The model under review builds one solid part; all positions refer to its coordinate system, in mm. Give positions to 0.01 mm unless a question says otherwise; leave off trailing zeros. Order: outer loops, then holes, each group sorted by start corner. A loop starts at its lowest first (then second) coordinate and runs counter-clockwise, first axis right, second up. Notation, with made-up numbers: (49.5, 56.5) - (65.5, 56.5) arc R25 cw to (65.5, 85.5) - close; hole circle Ø7 at (49, 64). An arc over 180 degrees is marked (long way). Use CSV: the item, a comma, the result in double quotes.
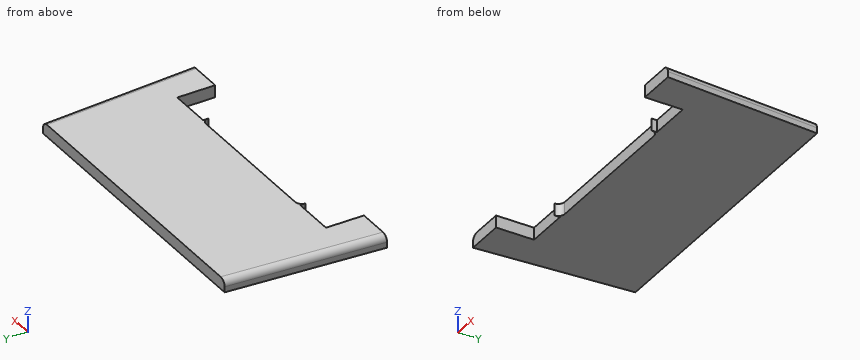
```python
from build123d import *

# Parameters (mm, degrees)
BOSS_EXTRUDE1_DEPTH = 25
FILLET1_R           = 13.5


with BuildPart() as part:
    # Sketch1 → Boss-Extrude1 (new body)
    with BuildSketch(Plane.XY):
        with BuildLine():
            Line((-251.2, -2), (-251.2, -80))
            Line((-251.2, -80), (-329.1, -80))
            Line((-329.1, -80), (-306.723420178, 240))
            Line((-306.723420178, 240), (306.723420178, 240))
            Line((306.723420178, 240), (329.1, -80))
            Line((329.1, -80), (251.2, -80))
            Line((251.2, -80), (251.2, -2))
            Line((251.2, -2), (163.8, -2))
            Line((163.8, -2), (163.8, -13))
            ThreePointArc((163.8, -13), (159.992388155, -3.807611845), (150.8, 0))
            Line((150.8, 0), (-150.8, 0))
            ThreePointArc((-150.8, 0), (-159.992388155, -3.807611845), (-163.8, -13))
            Line((-163.8, -13), (-163.8, -2))
            Line((-163.8, -2), (-251.2, -2))
        make_face()
    extrude(amount=BOSS_EXTRUDE1_DEPTH)

    # Fillet1
    fillet1_edges = [part.edges().sort_by_distance(p)[0] for p in [
        (317.911710089, 80, 25),
        (-317.911710089, 80, 25),
    ]]
    fillet(fillet1_edges, radius=FILLET1_R)


solid = part.part
```
Item 1: Take a section at C-C, the plane x = -210.5. Give the boundary of the cut face in (y, z).
Results list:
outline,"(-2, 0) - (240, 0) - (240, 25) - (-2, 25) - close"
Item 2: Clearance check with flat-ended pins moving along their axes: pin 1 (5 mm diameter, centred on y = 111, z = 15, fed in from -X); pin 2 (3.5 mm diameter, centred on y = -9.5, z = 10.5, fed in from -X); pin 3 (7.5 mm diameter, centred on x = 201.5, z = 16, fed in from -Y). State where each tip first meets the part, or that it passes through.
Results list:
pin 1,"stops at x = -315.77"
pin 2,"stops at x = -324.29"
pin 3,"stops at y = -2"
Item 3: Take a section at A-A, the plane z = 5.75. Give the boundary of the cut face in (x, y).
Results list:
outline,"(-329.1, -80) - (-251.2, -80) - (-251.2, -2) - (-163.8, -2) - (-163.8, -13) arc R13 cw to (-150.8, 0) - (150.8, 0) arc R13 cw to (163.8, -13) - (163.8, -2) - (251.2, -2) - (251.2, -80) - (329.1, -80) - (306.72, 240) - (-306.72, 240) - close"
Item 4: Take a section at B-B, the plane x = 55. Give the boundary of the cut face in (y, z).
Results list:
outline,"(0, 0) - (240, 0) - (240, 25) - (0, 25) - close"
Item 5: Wall thickness on L1, parallel to X at y = -34.5, z = 6.5; L2, parallel to Y at x = -146.5, z = 4.5; L3, parallel to Y at x = -191, z = 9.75: over which ranges is each line inside the solid? List them lowest first.
Results list:
L1,"x = -325.92 to -251.2, 251.2 to 325.92"
L2,"y = 0 to 240"
L3,"y = -2 to 240"
